```python
from build123d import *

# Parameters (mm, degrees)
CHAMFER1_SIZE      = 1
CUT_EXTRUDE1_REACH = 59.446
SKETCH3_R          = 2.5
FILLET1_R          = 2
CHAMFER2_SIZE      = 1
CHAMFER3_SIZE      = 0.5


with BuildPart() as part:
    # Sketch1 → Revolve1 (revolve)
    with BuildSketch(Plane.XY, mode=Mode.PRIVATE) as revolve1_sk:
        Polygon((-15, 0), (-15, 20), (-25, 20), (-25, 10), (-40, 10), (-40, 0), align=None)
    revolve(revolve1_sk.sketch.rotate(Axis((0, 0, 0), (0, 1, 0)), 270), axis=Axis((0, 0, 0), (0, 1, 0)))

    # Chamfer1
    chamfer1_edges = [part.edges().sort_by_distance(p)[0] for p in [
        (0, 20, 15),
    ]]
    chamfer(chamfer1_edges, length=CHAMFER1_SIZE)

    # Sketch3 → Cut-Extrude1 (cut, up to next)
    with BuildSketch(Plane(origin=(0, 10, 0), x_dir=(1, 0, 0), z_dir=(0, 1, 0)), mode=Mode.PRIVATE) as cut_extrude1_sk1:
        with Locations(Location((17.5, 30.310889132, 0), (0, 0, 270))):
            Circle(SKETCH3_R)
    cut_extrude1_tool1 = extrude(cut_extrude1_sk1.sketch, amount=-CUT_EXTRUDE1_REACH, mode=Mode.PRIVATE) & part.part
    # Sketch3 → Cut-Extrude1 (cut, up to next)
    with BuildSketch(Plane(origin=(0, 10, 0), x_dir=(1, 0, 0), z_dir=(0, 1, 0)), mode=Mode.PRIVATE) as cut_extrude1_sk2:
        with Locations(Location((30.310889132, -17.5, 0), (0, 0, 270))):
            Circle(SKETCH3_R)
    cut_extrude1_tool2 = extrude(cut_extrude1_sk2.sketch, amount=-CUT_EXTRUDE1_REACH, mode=Mode.PRIVATE) & part.part
    # Sketch3 → Cut-Extrude1 (cut, up to next)
    with BuildSketch(Plane(origin=(0, 10, 0), x_dir=(1, 0, 0), z_dir=(0, 1, 0)), mode=Mode.PRIVATE) as cut_extrude1_sk3:
        with Locations(Location((-17.5, -30.310889132, 0), (0, 0, 270))):
            Circle(SKETCH3_R)
    cut_extrude1_tool3 = extrude(cut_extrude1_sk3.sketch, amount=-CUT_EXTRUDE1_REACH, mode=Mode.PRIVATE) & part.part
    # Sketch3 → Cut-Extrude1 (cut, up to next)
    with BuildSketch(Plane(origin=(0, 10, 0), x_dir=(1, 0, 0), z_dir=(0, 1, 0)), mode=Mode.PRIVATE) as cut_extrude1_sk4:
        with Locations(Location((-30.310889132, 17.5, 0), (0, 0, 270))):
            Circle(SKETCH3_R)
    cut_extrude1_tool4 = extrude(cut_extrude1_sk4.sketch, amount=-CUT_EXTRUDE1_REACH, mode=Mode.PRIVATE) & part.part
    add(cut_extrude1_tool1.solids().sort_by_distance((17.5, 10, -30.310889))[0], mode=Mode.SUBTRACT)
    add(cut_extrude1_tool2.solids().sort_by_distance((30.310889, 10, 17.5))[0], mode=Mode.SUBTRACT)
    add(cut_extrude1_tool3.solids().sort_by_distance((-17.5, 10, 30.310889))[0], mode=Mode.SUBTRACT)
    add(cut_extrude1_tool4.solids().sort_by_distance((-30.310889, 10, -17.5))[0], mode=Mode.SUBTRACT)

    # Fillet1
    fillet1_edges = [part.edges().sort_by_distance(p)[0] for p in [
        (0, 10, 25),
    ]]
    fillet(fillet1_edges, radius=FILLET1_R)

    # Chamfer2
    chamfer2_edges = [part.edges().sort_by_distance(p)[0] for p in [
        (0, 0, 40),
        (0, 10, 40),
        (0, 20, 25),
    ]]
    chamfer(chamfer2_edges, length=CHAMFER2_SIZE)

    # Chamfer3
    chamfer3_edges = [part.edges().sort_by_distance(p)[0] for p in [
        (0, 0, 15),
    ]]
    chamfer(chamfer3_edges, length=CHAMFER3_SIZE)


solid = part.part
```
For this review, take the finished solid that the model builds, in its own axes (mm). A direction names the side the tool comes from. Round coordinates to 2 decimals unless told otherwise and drop trailing zeros. Write each loop counter-clockwise with the first axis right and the second up, starting at its lowest first coordinate (ties: lowest second). Pieces come first, ordered by that corner, then holes. Notation, with made-up numbers: (83, 52) -> (134, 52) arc R19 cw to (134, 77) -> close; hole circle Ø4 at (-28.75, 51). An arc over 180 degrees is marked (long way). Use one line per item in the form item = value.
Q1. Consider section B-B (z = 0). State the section outline as (x, y) points.
Resolved:
outline = (-40, 1) -> (-39, 0) -> (-15.5, 0) -> (-15, 0.5) -> (-15, 19) -> (-16, 20) -> (-24, 20) -> (-25, 19) -> (-25, 12) arc R2 cw to (-27, 10) -> (-39, 10) -> (-40, 9) -> close; (15, 0.5) -> (15.5, 0) -> (39, 0) -> (40, 1) -> (40, 9) -> (39, 10) -> (27, 10) arc R2 cw to (25, 12) -> (25, 19) -> (24, 20) -> (16, 20) -> (15, 19) -> close
Q2. The part is to be moulded in two halves that separate along Z. For faces 1 (the flat face through (-27, 10, 8)), 2 (the cylindrical face through (-32.75, 5.07, -18.04)), 3 (the cylindrical face through (39.05, 4.94, 8.67)), say which applies: released by +Z, released by -Z, zero draft, split by the parting line, or undercut.
Resolved:
face_1 = zero draft
face_2 = undercut
face_3 = split by the parting line
Q3. Machinability: for faces 4 (the cylindrical face through (-7.509, 15.451, -23.846)), 5 (the cylindrical face through (18.251, 5.07, -27.926)), which of the approach directions +Z, -Z, +X, -X, +Y, -Y give a long, thin tool a straight path to every point of the face, cutting with its end or side? Answer none if there is none.
Resolved:
face_4 = +Y
face_5 = +Y, -Y
Q4. Consider section C-C (y = 2.5). State the section outline as (x, z) points.
Resolved:
outline = circle Ø80 at (0, 0); hole circle Ø5 at (-30.31, -17.5); hole circle Ø5 at (-17.5, 30.31); hole circle Ø30 at (0, 0); hole circle Ø5 at (17.5, -30.31); hole circle Ø5 at (30.31, 17.5)
Q5. Clearance check with flat-ended pins moving along their axes: pin 1 Ø6 at (y, z) = (9.5, 7) entering from -X; pin 2 Ø12 at (x, z) = (4, -9) entering from +Y; pin 3 Ø3 at (x, z) = (-18, 27.5) entering from -Y; pin 4 Ø1.5 at (x, y) = (-4.5, 16.5) entering from +Z. State where each tip first meets the part, or that it passes through.
Resolved:
pin_1 = -39.8
pin_2 = 19.85
pin_3 = 0
pin_4 = 24.72
Q6. To check wall thickness, follow probe 1 along X at (y, z) = (12.5, 0); probe 2 along Y at (x, z) = (-13.5, 30.5); probe 3 along X at (y, z) = (10.5, -7). State the ranges of each line that lie inside material, in increasing order. Write a range as from..to.
Resolved:
probe_1 = -25..-15, 15..25
probe_2 = 0..10
probe_3 = -24.7..-13.27, 13.27..24.7
Q7. Consider section A-A (x = 0). State the section outline as (y, z) points, then the cut area to 3 significant figures.
Resolved:
outline = (0, -39) -> (1, -40) -> (9, -40) -> (10, -39) -> (10, -27) arc R2 cw to (12, -25) -> (19, -25) -> (20, -24) -> (20, -16) -> (19, -15) -> (0.5, -15) -> (0, -15.5) -> close; (0, 15.5) -> (0.5, 15) -> (19, 15) -> (20, 16) -> (20, 24) -> (19, 25) -> (12, 25) arc R2 cw to (10, 27) -> (10, 39) -> (9, 40) -> (1, 40) -> (0, 39) -> close
area = 697 mm²
